from build123d import *

# Parameters (mm, degrees)
SKETCH1_R           = 5
BOSS_EXTRUDE1_DEPTH = 10
SKETCH2_R           = 2.5
BOSS_EXTRUDE2_DEPTH = 15


with BuildPart() as part:
    # Sketch1 → Boss-Extrude1 (new body)
    with BuildSketch(Plane(origin=(0, 0, 0), x_dir=(1, 0, 0), z_dir=(0, 1, 0))):
        with BuildLine():
            Line((0, 6), (108, 6))
            ThreePointArc((108, 6), (114, 0), (108, -6))
            Line((108, -6), (0, -6))
            ThreePointArc((0, -6), (-6, 0), (0, 6))
        make_face()
        Circle(SKETCH1_R, mode=Mode.SUBTRACT)
        with Locations((42.5, 0)):
            Circle(SKETCH1_R, mode=Mode.SUBTRACT)
    extrude(amount=BOSS_EXTRUDE1_DEPTH)

    # Sketch2 → Boss-Extrude2 (add)
    with BuildSketch(Plane(origin=(0, 10, 0), x_dir=(1, 0, 0), z_dir=(0, 1, 0))):
        with Locations((108, 0)):
            Circle(SKETCH2_R)
    extrude(amount=BOSS_EXTRUDE2_DEPTH)


solid = part.part
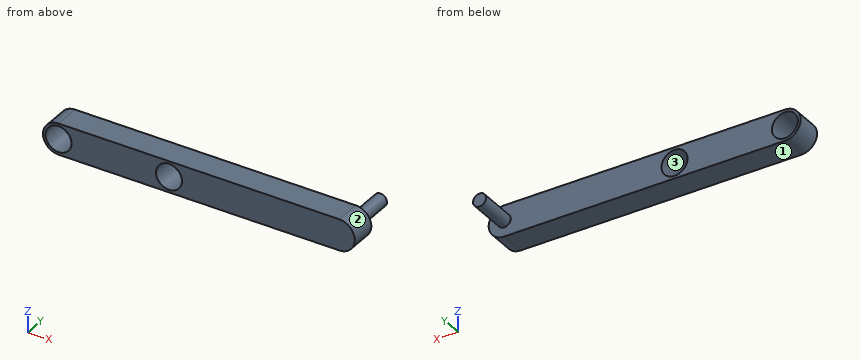
Could you check a few things on this model? Use its own coordinates, in mm. Face numbers are marked on the shaded views. Give positions to 0.01 mm unless a question says otherwise; leave off trailing zeros. Order: outer loops, then holes, each group sorted by start corner. A loop starts at its lowest first (then second) coordinate and runs counter-clockwise, first axis right, second up. Notation, with made-up numbers: (43, -12) - (81, -12) arc R21 cw to (81, 12) - close; hole circle Ø2 at (44, 16). An arc over 180 degrees is marked (long way). One line per item, written item: value. Start each with the question number.
1. For P1, Ø1, axis at y = 12, z = 2.5, coming from the -X side; P2, Ø5, axis at x = 81.5, z = -1, coming from the +Y side; P3, Ø3, axis at y = 18.5, z = -2, coming from the -X side; P4, Ø2, axis at x = 95, z = -3, coming from the -Y side, each with a flat end and sliding along its axis, tell me the tip position at first contact or that it passes through.
2. Imagine slicing it at C-C on y = 7. List the corners of the cut face in (x, z) for me.
3. Imagine slicing it at A-A on z = 0. List the corners of the cut face in (x, y) for me, plus the area to 4 significant figures.
4. Imagine slicing it at D-D on x = 91.5. List the corners of the cut face in (y, z) for me, plus the area to 3 significant figures.
5. Thinking about a two-plate mould opening in X: for the marked faces 1, 2 and 3, which applies, +X half, -X half, draft (parallel to the pull), parting line (faces both ways), or undercut?
6. If I drill on probe 1 along X at (y, z) = (7.25, 0); probe 2 along Z at (x, y) = (42.5, 4); probe 3 along X at (y, z) = (7.25, 2.5), over which ranges is the centre line in solid material (lowest first)?
7. Imagine slicing it at B-B on x = 39.5. List the corners of the cut face in (y, z) for me.
Values:
1. P1: x = 106.5
1. P2: y = 10
1. P3: x = 105.55
1. P4: y = 0
2. outline: (0, -6) - (108, -6) arc R6 ccw to (108, 6) - (0, 6) arc R6 ccw to start; hole circle Ø10 at (0, 0); hole circle Ø10 at (42.5, 0)
3. outline: (-6, 0) - (-5, 0) - (-5, 10) - (-6, 10) - close; (5, 0) - (37.5, 0) - (37.5, 10) - (5, 10) - close; (47.5, 0) - (114, 0) - (114, 10) - (110.5, 10) - (110.5, 25) - (105.5, 25) - (105.5, 10) - (47.5, 10) - close
3. area: 1,075 mm²
4. outline: (0, -6) - (10, -6) - (10, 6) - (0, 6) - close
4. area: 120 mm²
5. face 1: draft
5. face 2: +X half
5. face 3: undercut
6. probe 1: -6 to -5, 5 to 37.5, 47.5 to 114
6. probe 2: -6 to -5, 5 to 6
6. probe 3: -5.45 to -4.33, 4.33 to 38.17, 46.83 to 113.45
7. outline: (0, -6) - (10, -6) - (10, -4) - (0, -4) - close; (0, 4) - (10, 4) - (10, 6) - (0, 6) - close
